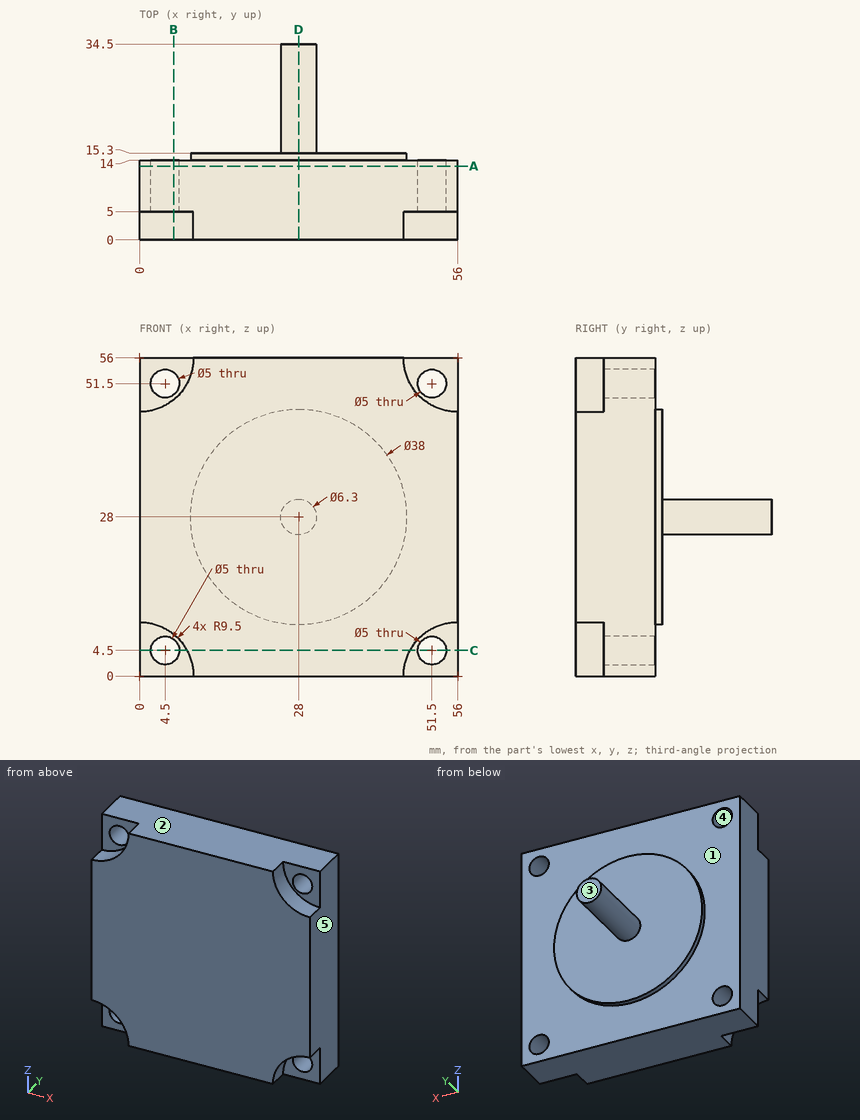
Drawing for the job (mm, zero at the part's lowest x, y, z). A direction names the side the tool comes from. Give positions to 0.01 mm unless a question says otherwise; leave off trailing zeros. Loops run counter-clockwise (first coordinate to the right, second up) from the corner with the lowest first, then second, coordinate; pieces in that order, holes last.
(1) Pin check, flat tips, straight feed: pin 1 (8 mm diameter, centred on y = 20.5, z = 33.5, fed in from +X); pin 2 (1 mm diameter, centred on x = 30, y = 30, fed in from -Z); pin 3 (3 mm diameter, centred on x = 51, z = 3, fed in from -Y). Stop position of each tip, or through.
Return value:
pin 1: stops at x = 30.77
pin 2: stops at z = 25.23
pin 3: stops at y = 5
(2) Band-saw the part on A-A (y = 13). Write the cut outline in (x, z).
Return value:
outline: (0, 0) - (56, 0) - (56, 56) - (0, 56) - close; hole circle Ø5 at (4.5, 4.5); hole circle Ø5 at (4.5, 51.5); hole circle Ø5 at (51.5, 4.5); hole circle Ø5 at (51.5, 51.5)
(3) Band-saw the part on C-C (z = 4.5). Write the cut outline in (x, y).
Return value:
outline: (0, 5) - (2, 5) - (2, 14) - (0, 14) - close; (7, 5) - (8.37, 5) - (8.37, 0) - (47.63, 0) - (47.63, 5) - (49, 5) - (49, 14) - (7, 14) - close; (54, 5) - (56, 5) - (56, 14) - (54, 14) - close
(4) Pull direction X, two halves, no side cores. Call the marked faces 3, 4 and 5: pulls with the +X half, pulls with the -X half, needs draft (parallel to the pull), parting line crosses it, or undercut.
Return value:
face 3: needs draft
face 4: undercut
face 5: pulls with the +X half
(5) Band-saw the part on B-B (x = 6). Write the cut outline in (y, z), and give its area (3 significant figures).
Return value:
outline: (0, 7.37) - (5, 7.37) - (5, 6.5) - (14, 6.5) - (14, 49.5) - (5, 49.5) - (5, 48.63) - (0, 48.63) - close; (5, 0) - (14, 0) - (14, 2.5) - (5, 2.5) - close; (5, 53.5) - (14, 53.5) - (14, 56) - (5, 56) - close
area: 638 mm2
(6) Band-saw the part on D-D (x = 28). Write the cut outline in (y, z), and give its area (3 significant figures).
Return value:
outline: (0, 0) - (14, 0) - (14, 9) - (15.3, 9) - (15.3, 24.85) - (34.5, 24.85) - (34.5, 31.15) - (15.3, 31.15) - (15.3, 47) - (14, 47) - (14, 56) - (0, 56) - close
area: 954 mm2
(7) 3-axis set-ups, long thin cutter, end or side, ignore diameter. For the marked faces 1 and 2: which of +Z, -Z, +X, -X, +Y, -Y reach the whole face in a straight line?
Return value:
face 1: +Y
face 2: +Z, +X, -X, +Y, -Y
(8) Drill centre lines: line 1 along X through (y, z) = (10, 51.5); line 2 along Z through (x, y) = (6.5, 11); line 3 along Z through (x, y) = (4, 12.5). Where is each one in solid material? Low to high.
Return value:
line 1: x = 0 to 2, 7 to 49, 54 to 56
line 2: z = 0 to 3, 6 to 50, 53 to 56
line 3: z = 0 to 2.05, 6.95 to 49.05, 53.95 to 56
